Check sheet for the modelled part. Datum: model origin and axes. Units: mm. Face numbers are marked on the shaded views. A direction names the side the tool comes from. Coordinates: 2 decimals unless noted, no trailing zeros. Loops run counter-clockwise (first coordinate to the right, second up) from the corner with the lowest first, then second, coordinate; pieces in that order, holes last. Notation, with made-up numbers: (-7, -24.75) -> (43, -24.75) arc R13 cw to (43, -17.75) -> close; hole circle Ø6 at (-3.75, -6). An arc over 180 degrees is marked (long way). Use CSV: the item, a comma, the result in double quotes. Start each with the question number.
1. Sectioned sample at D-D, the plane x = 41. Record the cut outline in (y, z), and give its area (3 significant figures).
2. Release check for a two-part mould opening along Y. For the marked faces 3, 4 and 5 record: pulls with the +Y half, pulls with the -Y half, needs draft (parallel to the pull), parting line crosses it, or undercut.
3. Gauge pin test, flat ends, axial feed: pin 1 (3.5 mm diameter, centred on y = -24, z = 28, fed in from +X); pin 2 (6 mm diameter, centred on x = -3, y = -24, fed in from +Z). Record the tip position at first contact, or that the pin passes through.
4. Sectioned sample at B-B, the plane y = 0. Record the cut outline in (x, z), and give its area (3 significant figures).
5. Sectioned sample at A-A, the plane z = 28. Record the cut outline in (x, y), and give its area (3 significant figures).
6. Set-up check for the marked faces 1 and 2: record each of +Z, -Z, +X, -X, +Y, -Y from which the full face is reachable in a straight line by a thin tool's end or side.
7. Thickness scan on L1, parallel to Y at x = -97, z = 28; L2, parallel to Y at x = 20, z = 12.5; L3, parallel to X at y = 35, z = 33.5. Record the ranges inside material, lowest first.
8. Sectioned sample at C-C, the plane z = 8.5. Record the cut outline in (x, y).
```python
from build123d import *

# Parameters (mm, degrees)
SKETCH_2_W          = 200
SKETCH_2_H          = 80
EXTRUDE_1_DEPTH     = 56
SKETCH_3_W          = 192
SKETCH_3_H          = 72
CUT_EXTRUDE_1_DEPTH = 52
SKETCH_6_R          = 13
CUT_EXTRUDE_2_DEPTH = 4
SKETCH_8_R          = 3
CUT_EXTRUDE_3_DEPTH = 10


with BuildPart() as part:
    # 草图2 → 凸台-拉伸1 (new body)
    with BuildSketch(Plane.XY):
        Rectangle(SKETCH_2_W, SKETCH_2_H)
    extrude(amount=EXTRUDE_1_DEPTH)

    # 草图3 → 切除-拉伸1 (cut)
    with BuildSketch(Plane.XY.offset(56)):
        Rectangle(SKETCH_3_W, SKETCH_3_H)
    extrude(amount=-CUT_EXTRUDE_1_DEPTH, mode=Mode.SUBTRACT)

    # 草图6 → 切除-拉伸2 (cut)
    with BuildSketch(Plane.ZY.offset(100)):
        with Locations((28, 0)):
            Circle(SKETCH_6_R)
    extrude(amount=-CUT_EXTRUDE_2_DEPTH, mode=Mode.SUBTRACT)

    # 草图8 → 切除-拉伸3 (cut)
    with BuildSketch(Plane(origin=(100, 0, 0), x_dir=(0, 0, -1), z_dir=(1, 0, 0))):
        with Locations((-28, 24)):
            Circle(SKETCH_8_R)
        with Locations((-28, -24)):
            Circle(SKETCH_8_R)
    extrude(amount=-CUT_EXTRUDE_3_DEPTH, mode=Mode.SUBTRACT)


solid = part.part
```
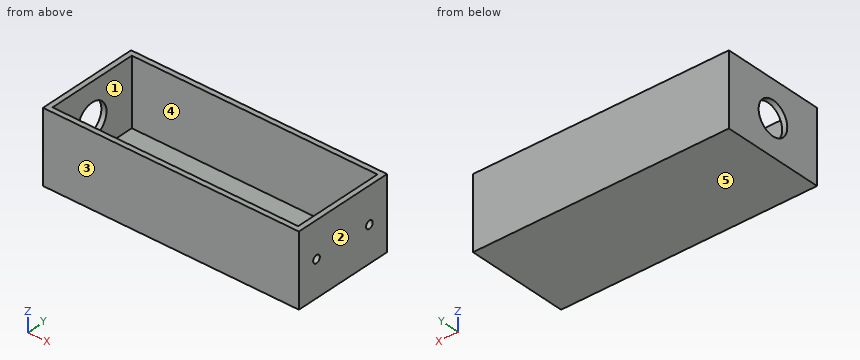
Completed:
1,outline,"(-40, 0) -> (40, 0) -> (40, 56) -> (36, 56) -> (36, 4) -> (-36, 4) -> (-36, 56) -> (-40, 56) -> close"
1,area,"736 mm²"
2,face 3,"pulls with the -Y half"
2,face 4,"undercut"
2,face 5,"needs draft"
3,pin 1,"x = -96"
3,pin 2,"z = 4"
4,outline,"(-100, 0) -> (100, 0) -> (100, 56) -> (96, 56) -> (96, 4) -> (-96, 4) -> (-96, 15) -> (-100, 15) -> close; (-100, 41) -> (-96, 41) -> (-96, 56) -> (-100, 56) -> close"
4,area,"1,110 mm²"
5,outline,"(-100, -40) -> (100, -40) -> (100, -27) -> (96, -27) -> (96, -36) -> (-96, -36) -> (-96, -13) -> (-100, -13) -> close; (-100, 13) -> (-96, 13) -> (-96, 36) -> (96, 36) -> (96, 27) -> (100, 27) -> (100, 40) -> (-100, 40) -> close; (96, -21) -> (100, -21) -> (100, 21) -> (96, 21) -> close"
5,area,"2,020 mm²"
6,face 1,"+Z"
6,face 2,"+Z, -Z, +X, +Y, -Y"
7,L1,"-40 to -13, 13 to 40"
7,L2,"-40 to -36, 36 to 40"
7,L3,"-100 to -96, 96 to 100"
8,outline,"(-100, -40) -> (100, -40) -> (100, 40) -> (-100, 40) -> close; hole (-96, -36) -> (96, -36) -> (96, 36) -> (-96, 36) -> close"
